Build history of the part. All positions in model axes, mm. A direction names the side the tool comes from. Coordinates: 2 decimals unless noted, no trailing zeros. Order: outer loops, then holes, each group sorted by start corner. A loop starts at its lowest first (then second) coordinate and runs counter-clockwise, first axis right, second up. Notation, with made-up numbers: M 79,6 L 107,6 A17 cw 107,32 Z; hole C -5.5,-32.75 d4. An arc over 180 degrees is marked long. Use a Markdown table: item, result. Add a question column.
from build123d import *

# Parameters (mm, degrees)
SKETCH1_W           = 38.1
SKETCH1_H           = 177.8
BOSS_EXTRUDE1_DEPTH = 3.175
SKETCH2_W           = 3.175
SKETCH2_H           = 12.7
SKETCH2_H_2         = 9.525
SKETCH2_W_2         = 12.809265573
SKETCH2_H_3         = 3.175
CUT_EXTRUDE1_DEPTH  = 3.175


with BuildPart() as part:
    # Sketch1 → Boss-Extrude1 (new body)
    with BuildSketch(Plane(origin=(0, 0, 0), x_dir=(1, 0, 0), z_dir=(0, 1, 0))):
        Rectangle(SKETCH1_W, SKETCH1_H)
    extrude(amount=BOSS_EXTRUDE1_DEPTH)

    # Sketch2 → Cut-Extrude1 (cut)
    with BuildSketch(Plane(origin=(0, 3.175, 0), x_dir=(1, 0, 0), z_dir=(0, 1, 0))):
        Polygon((-6.35, 88.9), (-6.35, 85.725), (-15.875, 85.725), (-15.875, 60.325), (-19.05, 60.325), (-19.05, 88.9), (-15.875, 88.9), align=None)
        with Locations((-17.4625, 15.875)):
            Rectangle(SKETCH2_W, SKETCH2_H)
        with Locations((-17.4625, 41.275)):
            Rectangle(SKETCH2_W, SKETCH2_H)
        with Locations((-17.4625, -9.525)):
            Rectangle(SKETCH2_W, SKETCH2_H)
        with Locations((-17.4625, -34.925)):
            Rectangle(SKETCH2_W, SKETCH2_H)
        with Locations((-17.4625, -60.325)):
            Rectangle(SKETCH2_W, SKETCH2_H)
        with Locations((-17.4625, -84.1375)):
            Rectangle(SKETCH2_W, SKETCH2_H_2)
        with Locations((12.645367214, 87.3125)):
            Rectangle(SKETCH2_W_2, SKETCH2_H_3)
    extrude(amount=-CUT_EXTRUDE1_DEPTH, mode=Mode.SUBTRACT)


solid = part.part
(1) Drill centre lines: line 1 along Z through (x, y) = (13, 1.25) (3 decimals); line 2 along X through (y, z) = (1.15, 57) (3 decimals). Where is each one in solid material? Low to high. Write a range as from..to.
(2) Slice it at B-B on x = 14. Give the cut face in (y, z) (3 decimals), and give its area (3 significant figures).
(3) Mould opens along Z. For faces 1 (the flat face through (-17, 2, -34.925)), 2 (the flat face through (-6.35, 2, -87)), 3 (the flat face through (-17, 2, 79.375)) say: released by +Z, released by -Z, zero draft, split by the parting line, or undercut.
(4) Which spindle directions (+Z, -Z, +X, -X, +Y, -Y) get a long thin tool onto all of the face, cutting with end or side? Do faces 4 (the flat face through (-19.05, 2, -28)), 5 (the flat face through (0, 3.175, -1)), 6 (the flat face through (6.241, 2, -87)), 7 (the flat face through (-17, 2, 41.275)), 8 (the flat face through (-15.875, 2, -73)). Say none if no direction does.
(5) Drop flat-ended pins along their axis: P1, Ø1, axis at x = -16.5, y = 2, coming from the +Z side (3 decimals); P2, Ø1, axis at y = 2, z = -14, coming from the -X side (3 decimals); P3, Ø1.6, axis at x = -17, y = 1.5, coming from the -Z side (3 decimals). Give the stop position or say it passes through.
(6) Slice it at C-C on z = 31.5. Give the cut face in (x, y) (3 decimals), and give its area (3 significant figures).
Solutions:
| question | item | result |
|---|---|---|
| 1 | line 1 | -85.725..88.9 |
| 1 | line 2 | -15.875..19.05 |
| 2 | outline | M 0,-85.725 L 3.175,-85.725 L 3.175,88.9 L 0,88.9 Z |
| 2 | area | 554 mm² |
| 3 | face 1 | undercut |
| 3 | face 2 | zero draft |
| 3 | face 3 | released by +Z |
| 4 | face 4 | +Z, -Z, -X, +Y, -Y |
| 4 | face 5 | +Z, -Z, +X, -X, +Y |
| 4 | face 6 | -Z, +X, +Y, -Y |
| 4 | face 7 | -X, +Y, -Y |
| 4 | face 8 | -Z, -X, +Y, -Y |
| 5 | P1 | z = 79.375 |
| 5 | P2 | x = -15.875 |
| 5 | P3 | z = -60.325 |
| 6 | outline | M -15.875,0 L 19.05,0 L 19.05,3.175 L -15.875,3.175 Z |
| 6 | area | 111 mm² |
